The figure shows three views and two pictorial views of one solid part (mm, origin at its lowest corner). Answer the questions. Give positions to 0.01 mm unless a question says otherwise; leave off trailing zeros. Loops run counter-clockwise (first coordinate to the right, second up) from the corner with the lowest first, then second, coordinate; pieces in that order, holes last.
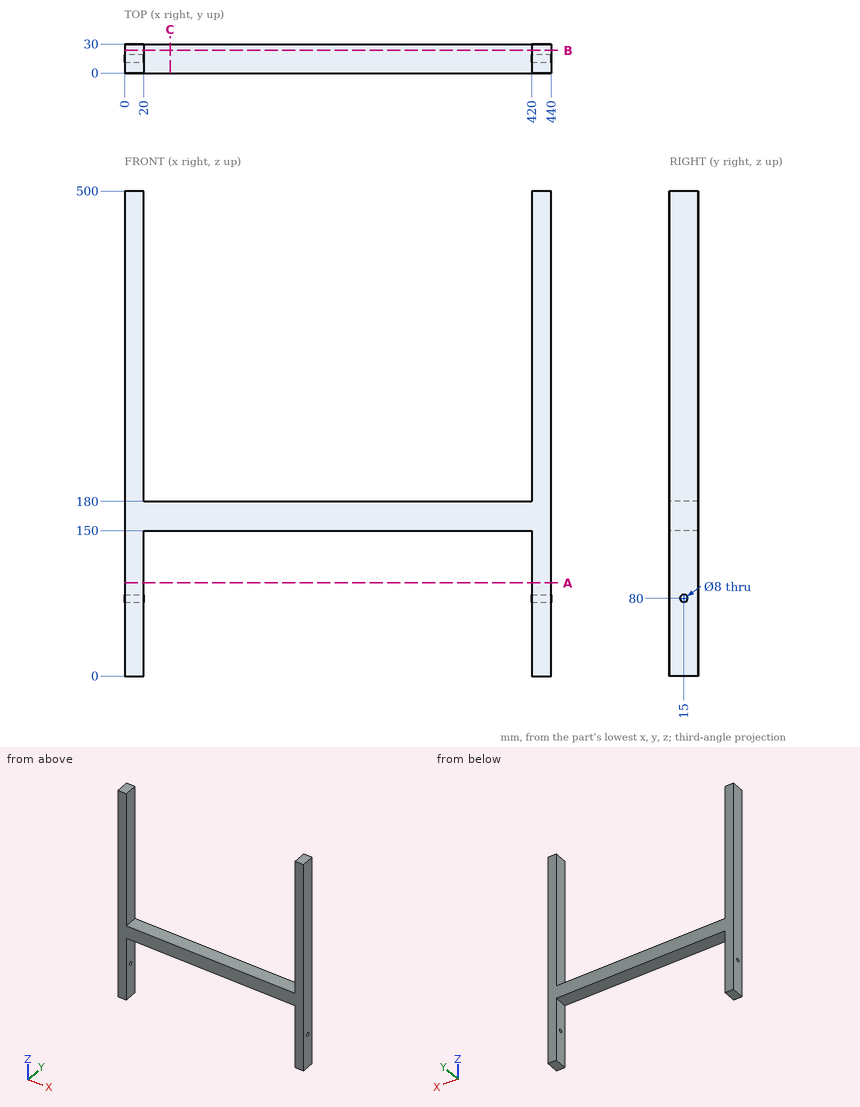
Q1. Given pin 1 (5 mm diameter, centred on y = 15, z = 80, fed in from +X); pin 2 (8 mm diameter, centred on x = 156.5, y = 14.5, fed in from -Z), each flat-ended and moving along its own axis, determine where each tip first touches the part or whether it passes through.
Q2. Section C-C on x = 47 is taken. Give the vertices of the cut face in (y, z), plus the area to 3 significant figures.
Q3. Section A-A on z = 96 is taken. Give the vertices of the cut face in (x, y).
Q4. Section B-B on y = 23.5 is taken. Give the vertices of the cut face in (x, z).
Q5. Consider line 1 along Z through (x, y) = (5.25, 15); line 2 along X through (y, z) = (22.75, 285); line 3 along Y through (x, z) = (426.75, 80). Determine where each line is inside the solid, lowest interval first.
Check result:
1. pin 1: passes through
1. pin 2: stops at z = 150
2. outline: (0, 150) - (30, 150) - (30, 180) - (0, 180) - close
2. area: 900 mm2
3. outline: (0, 0) - (20, 0) - (20, 30) - (0, 30) - close; (420, 0) - (440, 0) - (440, 30) - (420, 30) - close
4. outline: (0, 0) - (20, 0) - (20, 150) - (420, 150) - (420, 0) - (440, 0) - (440, 500) - (420, 500) - (420, 180) - (20, 180) - (20, 500) - (0, 500) - close
5. line 1: z = 0 to 76, 84 to 500
5. line 2: x = 0 to 20, 420 to 440
5. line 3: y = 0 to 11, 19 to 30
